For this review, take the finished solid that the model builds, in its own axes (mm). A direction names the side the tool comes from. Coordinates: 2 decimals unless noted, no trailing zeros. Order: outer loops, then holes, each group sorted by start corner. A loop starts at its lowest first (then second) coordinate and runs counter-clockwise, first axis right, second up. Notation, with made-up numbers: (-7, -18) - (48, -18) arc R8 cw to (48, -3) - close; hole circle Ø4 at (32, 4.25). An arc over 180 degrees is marked (long way). One line per item, written item: value. Start each with the question number.
(1) To check wall thickness, follow line 1 along Z through (x, y) = (0.5, -1); line 2 along Y through (x, z) = (-1.25, -5.25); line 3 along X through (y, z) = (-1.75, 7.25). State the ranges of each line that lie inside material, in increasing order.
(2) Clearance check with a flat-ended pin moving along its axis: pin 1 (3 mm diameter, centred on x = -2.5, z = -6.5, fed in from -Y). State where the tip first meets the part, or that it passes through.
(3) For faces 1 (the flat face through (0, 0, -8)), 2 (the flat face through (1.3, -1.3, 6)), list the 3-axis set-ups (+Z, -Z, +X, -X, +Y, -Y) from which the entire face can be reached by the end or side of a thin tool; tool diameter is ignored.
(4) Consider section A-A on z = 1.25. Write out the cut boundary in (x, y).
Autodesk Inventor part; units mm, degrees
ref_plane "YZ Plane" through (0, 0, 0) normal (1, 0, 0) x (0, 1, 0)
ref_plane "XZ Plane" through (0, 0, 0) normal (0, 1, 0) x (-1, 0, 0)
ref_plane "XY Plane" through (0, 0, 0) normal (0, 0, 1) x (1, 0, 0)
sketch "スケッチ1" plane through (0, 0, 0) normal (0, 0, 1) x (1, 0, 0)
  circle A0 centre (0, 0) radius 1.5
  dimension "d0" = 3
extrude "押し出し1" add sketch "スケッチ1" along normal blind 6
sketch "スケッチ2" plane through (0, 0, 6) normal (0, 0, 1) x (1, 0, 0)
  circle A0 centre (0, 0) radius 1.5
  circle A1 centre (0, 0) radius 3
  dimension "d3" = 6
extrude "押し出し2" add sketch "スケッチ2" along normal blind 2 contours A0 | A1
fillet "フィレット1" radius 2 1 edges at (-3, 0, 8)
thread "ねじ1"
sketch "スケッチ3" plane through (0, 0, 0) normal (0, 0, -1) x (-1, 0, 0)
  circle A0 centre (0, 0) radius 1.5
extrude "押し出し3" add sketch "スケッチ3" along normal blind 2
sketch "スケッチ4" plane through (0, 0, -2) normal (0, 0, -1) x (-1, 0, 0)
  circle A0 centre (0, 0) radius 1.5
extrude "押し出し4" add sketch "スケッチ4" along normal blind 2
sketch "スケッチ5" plane through (0, 0, -4) normal (0, 0, -1) x (-1, 0, 0)
  circle A0 centre (0, 0) radius 1.5
extrude "押し出し5" add sketch "スケッチ5" along normal blind 4
properties part number "SB　14mmなべネジ" material "Steel, Mild"
Geometry check:
1. line 1: z = -8 to 8
1. line 2: y = -0.83 to 0.83
1. line 3: x = -1.87 to 1.87
2. pin 1: stops at y = -1.12
3. face 1: -Z, +X, -X, +Y, -Y
3. face 2: -Z
4. outline: circle Ø3 at (0, 0)
